Answer from the drawing. Dimensions are ordinates in mm from the lowest x, y and z of the part. A direction names the side the tool comes from. Coordinates: 2 decimals unless noted, no trailing zeros. Order: outer loops, then holes, each group sorted by start corner. A loop starts at its lowest first (then second) coordinate and runs counter-clockwise, first axis right, second up. Notation, with made-up numbers: M 67,5.25 L 77,5.25 A34 ccw 77,37.25 Z; hole C 1,83.25 d10. An arc over 180 degrees is marked long. Write each question's results on one line, items separated by ' | '.
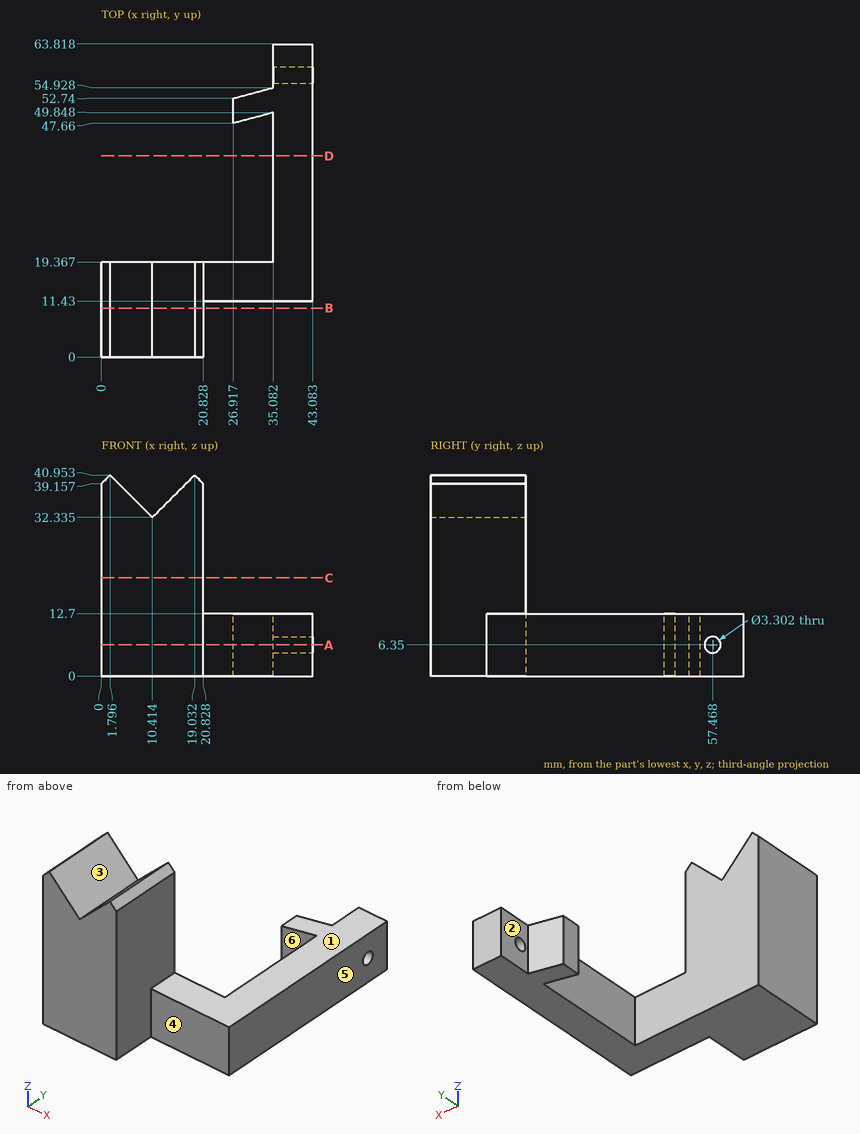
(1) The part is cut by section C-C, the plane z = 20. Write down the section's boundary in (x, y), then the cut area to 3 significant figures.
Conclusion:
outline: M 0,0 L 20.83,0 L 20.83,19.37 L 0,19.37 Z | area: 403 mm²
(2) The part is cut by section D-D, the plane y = 41. Write down the section's boundary in (x, z), then the cut area to 3 significant figures.
Conclusion:
outline: M 35.08,0 L 43.08,0 L 43.08,12.7 L 35.08,12.7 Z | area: 102 mm²
(3) Given pin 1 (6.5 mm diameter, centred on x = 36, z = 6, fed in from -Y); pin 2 (10.5 mm diameter, centred on x = 19, z = 19, fed in from +Y); pin 3 (8 mm diameter, centred on x = 25.5, y = 54.5, fed in from +Z), each flat-ended and moving along its own axis, determine where each tip first touches the part or whether it passes through.
Conclusion:
pin 1: y = 11.43 | pin 2: y = 19.37 | pin 3: z = 12.7
(4) The part is cut by section A-A, the plane z = 6.35. Write down the section's boundary in (x, y).
Conclusion:
outline: M 0,0 L 20.83,0 L 20.83,11.43 L 43.08,11.43 L 43.08,55.82 L 35.08,55.82 L 35.08,54.93 L 26.92,52.74 L 26.92,47.66 L 35.08,49.85 L 35.08,19.37 L 0,19.37 Z; M 35.08,59.12 L 43.08,59.12 L 43.08,63.82 L 35.08,63.82 Z
(5) The part is cut by section B-B, the plane y = 10. Write down the section's boundary in (x, z) (1 decimal).
Conclusion:
outline: M 0,0 L 20.8,0 L 20.8,39.2 L 19,41 L 10.4,32.3 L 1.8,41 L 0,39.2 Z
(6) The mould has two halves that part along Y. Classify the marked faces 4, 5 and 6: pulls with the +Y half, pulls with the -Y half, needs draft (parallel to the pull), parting line crosses it, or undercut.
Conclusion:
face 4: pulls with the -Y half | face 5: needs draft | face 6: undercut
(7) For the marked faces 1, 2 and 3, determine the directions among +Z, -Z, +X, -X, +Y, -Y from which every point of the face is accessible in a straight line to the end or side of a thin tool.
Conclusion:
face 1: +Z, +X, +Y, -Y | face 2: +Z, -Z, -X, +Y | face 3: +Z, +Y, -Y
(8) Straight lines are drawn through the part: line 1 (X direction, y = 42.5, z = 11); line 2 (X direction, y = 9.5, z = 23.5); line 3 (Y direction, x = 5, z = 4). For each, find the intervals that lie inside material, in ascending order.
Conclusion:
line 1: 35.08 to 43.08 | line 2: 0 to 20.83 | line 3: 0 to 19.37
